```python
from build123d import *

# Parameters (mm, degrees)
F0_R     = 6
F0_R_2   = 5
F0_R_3   = 5.872705
F1_DEPTH = 20
F2_DEPTH = 40


with BuildPart() as f1:
    # F0 (on Top) → F1 (new body)
    with BuildSketch(Plane.XY):
        with BuildLine():
            Line((167.5, 105), (-167.5, 105))
            Line((-167.5, 105), (-167.5, -105))
            Line((-167.5, -105), (-35, -105))
            Line((-35, -105), (-35, 0))
            ThreePointArc((-35, 0), (0, 35), (35, 0))
            Line((35, 0), (35, -105))
            Line((35, -105), (167.5, -105))
            Line((167.5, -105), (167.5, 105))
        make_face()
        with Locations((-142.5, -80)):
            Circle(F0_R, mode=Mode.SUBTRACT)
        with Locations((-60.621778, -35)):
            Circle(F0_R, mode=Mode.SUBTRACT)
        with Locations((142.5, -80)):
            Circle(F0_R, mode=Mode.SUBTRACT)
        with Locations((60.621778, -35)):
            Circle(F0_R, mode=Mode.SUBTRACT)
        with Locations((110, -35)):
            Circle(F0_R_2, mode=Mode.SUBTRACT)
        with Locations((-110, 35)):
            Circle(F0_R_2, mode=Mode.SUBTRACT)
        with Locations((-70, 0)):
            Circle(F0_R, mode=Mode.SUBTRACT)
        with Locations((-142.5, 80)):
            Circle(F0_R_3, mode=Mode.SUBTRACT)
        with Locations((-35, 60.621778)):
            Circle(F0_R, mode=Mode.SUBTRACT)
        with Locations((70, 0)):
            Circle(F0_R, mode=Mode.SUBTRACT)
        with Locations((35, 60.621778)):
            Circle(F0_R, mode=Mode.SUBTRACT)
        with Locations((0, 70)):
            Circle(F0_R, mode=Mode.SUBTRACT)
        with Locations((142.5, 80)):
            Circle(F0_R, mode=Mode.SUBTRACT)
    extrude(amount=F1_DEPTH)

    # F0 (on Top) → F2 (join)
    with BuildSketch(Plane.XY):
        with Locations((-110, 35)):
            Circle(F0_R_2)
        with Locations((110, -35)):
            Circle(F0_R_2)
    extrude(amount=F2_DEPTH)


solid = f1.part
```
Check sheet for the modelled part. Datum: model origin and axes. Units: mm. A direction names the side the tool comes from. Round coordinates to 2 decimals unless told otherwise and drop trailing zeros. Order: outer loops, then holes, each group sorted by start corner. A loop starts at its lowest first (then second) coordinate and runs counter-clockwise, first axis right, second up. Notation, with made-up numbers: M 52.5,22 L 98.5,22 A22 cw 98.5,48 Z; hole C -20.75,27.25 d11. An arc over 180 degrees is marked long. Answer in a Markdown table with one row per item.
(1) Section check C-C on y = -35. Record the boundary of the cut face in (x, z).
Findings:
| item | result |
|---|---|
| outline | M -167.5,0 L -66.62,0 L -66.62,20 L -167.5,20 Z; M -54.62,0 L -35,0 L -35,20 L -54.62,20 Z; M 35,0 L 54.62,0 L 54.62,20 L 35,20 Z; M 66.62,0 L 167.5,0 L 167.5,20 L 115,20 L 115,40 L 105,40 L 105,20 L 66.62,20 Z |
(2) Material ranges on line 1 along Y through (x, z) = (-142, 14); line 2 along Y through (x, z) = (142.5, 7.75); line 3 along X through (y, z) = (-82, 15.5), recorded low to high. Write a range as from..to.
Findings:
| item | result |
|---|---|
| line 1 | y = -105..-85.98, -74.02..74.15, 85.85..105 |
| line 2 | y = -105..-86, -74..74, 86..105 |
| line 3 | x = -167.5..-148.16, -136.84..-35, 35..136.84, 148.16..167.5 |
(3) Gauge pin test, flat ends, axial feed: pin 1 (7 mm diameter, centred on x = -35, y = 60.62, fed in from -Z); pin 2 (8 mm diameter, centred on x = 78.5, y = 13, fed in from +Z); pin 3 (1 mm diameter, centred on x = -113.5, z = 26.5, fed in from +Y). Record the tip position at first contact, or that the pin passes through.
Findings:
| item | result |
|---|---|
| pin 1 | passes through |
| pin 2 | stops at z = 20 |
| pin 3 | stops at y = 39 |
(4) Section check B-B on x = -70. Record the boundary of the cut face in (y, z), plus the area to 3 significant figures.
Findings:
| item | result |
|---|---|
| outline | M -105,0 L -6,0 L -6,20 L -105,20 Z; M 6,0 L 105,0 L 105,20 L 6,20 Z |
| area | 3,960 mm^2 |
(5) Draft check along Y on faces 4 (the cylindrical face through (-35.78, 66.57, 9.86)), 5 (the flat face through (-102, -105, 10)), 6 (the flat face through (-40, 1, 0)), 7 (the cylindrical face through (-55.08, -37.3, 9.86)). Enter one of: +Y half, -Y half, draft (parallel to the pull), parting line (faces both ways), or undercut.
Findings:
| item | result |
|---|---|
| face 4 | undercut |
| face 5 | -Y half |
| face 6 | draft |
| face 7 | undercut |
(6) Section check D-D on z = 34. Record the boundary of the cut face in (x, y), plus the area to 3 significant figures.
Findings:
| item | result |
|---|---|
| outline | C -110,35 d10; C 110,-35 d10 |
| area | 157 mm^2 |
(7) Section check A-A on y = 70. Record the boundary of the cut face in (x, z), plus the area to 3 significant figures.
Findings:
| item | result |
|---|---|
| outline | M -167.5,0 L -6,0 L -6,20 L -167.5,20 Z; M 6,0 L 167.5,0 L 167.5,20 L 6,20 Z |
| area | 6,460 mm^2 |
(8) Set-up check for faces 1 (the cylindrical face through (138.08, -75.94, 9.86)), 2 (the cylindrical face through (-105.23, 36.5, 29.86)), 3 (the flat face through (35, -52, 10)): record each of +Z, -Z, +X, -X, +Y, -Y from which the full face is reachable in a straight line by a thin tool's end or side.
Findings:
| item | result |
|---|---|
| face 1 | +Z, -Z |
| face 2 | +Z |
| face 3 | +Z, -Z, -Y |
